Verification items for the finished model (mm, model axes). A direction names the side the tool comes from. Give positions to 0.01 mm unless a question says otherwise; leave off trailing zeros. Loops run counter-clockwise (first coordinate to the right, second up) from the corner with the lowest first, then second, coordinate; pieces in that order, holes last. Notation, with made-up numbers: M -34.75,-10 L -9.75,-10 A31 cw -9.75,20 Z; hole C -40,-7 d1. An arc over 180 degrees is marked long. Use a Markdown table: item, result.
from build123d import *

# Parameters (mm, degrees)
BOSS_EXTRUDE1_DEPTH = 150
SKETCH2_W           = 12.7
SKETCH2_H           = 24.13
CUT_EXTRUDE1_DEPTH  = 156.216502449
SKETCH3_W           = 149.993973466
SKETCH3_H           = 14.75620072
BOSS_EXTRUDE2_DEPTH = 3.55599999
SKETCH4_W           = 3.55599999
SKETCH4_H           = 13.202768596
CUT_EXTRUDE2_DEPTH  = 152.137564539
DRAFT1_START        = -153.930973466
DRAFT1_DEPTH        = 149.993973466
DRAFT2_START        = -153.937
DRAFT2_DEPTH        = 150
FILLET1_R           = 0.76200009
FILLET2_R           = 1.98120009
FILLET3_R           = 2.54


# Read off the part's stored shape, not the designer's step: Draft1, Draft2
with BuildPart() as part:
    # Sketch1 → Boss-Extrude1 (new body)
    with BuildSketch(Plane(origin=(-3.937, 0, 0), x_dir=(0, 0, -1), z_dir=(1, 0, 0))):
        with BuildLine():
            Line((2.311399989, 16.37657286), (2.311399989, -16.37657286))
            ThreePointArc((2.311399989, -16.37657286), (0.354826715, -15.481038557), (-1.770730805, -15.815950332))
            ThreePointArc((-1.770730805, -15.815950332), (-3.400639082, -15.955235788), (-4.710462095, -14.975253591))
            Line((-4.710462095, -14.975253591), (-5.7404, -15.627692517))
            ThreePointArc((-5.7404, -15.627692517), (-3.73586423, -17.127444277), (-1.241474216, -16.914283663))
            ThreePointArc((-1.241474216, -16.914283663), (0.188944014, -16.688900954), (1.505642365, -17.291560998))
            ThreePointArc((1.505642365, -17.291560998), (2.81343034, -17.487614789), (3.53059999, -16.37657286))
            Line((3.53059999, -16.37657286), (3.53059999, 16.37657286))
            ThreePointArc((3.53059999, 16.37657286), (2.81343034, 17.487614789), (1.505642365, 17.291560998))
            ThreePointArc((1.505642365, 17.291560998), (0.188944014, 16.688900954), (-1.241474216, 16.914283663))
            ThreePointArc((-1.241474216, 16.914283663), (-3.73586423, 17.127444277), (-5.7404, 15.627692517))
            Line((-5.7404, 15.627692517), (-4.710462095, 14.975253591))
            ThreePointArc((-4.710462095, 14.975253591), (-3.400639082, 15.955235788), (-1.770730805, 15.815950332))
            ThreePointArc((-1.770730805, 15.815950332), (0.354826715, 15.481038557), (2.311399989, 16.37657286))
        make_face()
    extrude(amount=-BOSS_EXTRUDE1_DEPTH)

    # Sketch2 → Cut-Extrude1 (cut, through all)
    with BuildSketch(Plane(origin=(0, 0, -3.53059999), x_dir=(-1, 0, 0), z_dir=(0, 0, -1))):
        with Locations((10.287, 0)):
            Rectangle(SKETCH2_W, SKETCH2_H)
    extrude(amount=-CUT_EXTRUDE1_DEPTH, mode=Mode.SUBTRACT)

    # Sketch3 → Boss-Extrude2 (add)
    with BuildSketch(Plane.XY.offset(-2.311399989)):
        with Locations((-78.933986733, 0)):
            Rectangle(SKETCH3_W, SKETCH3_H)
    extrude(amount=BOSS_EXTRUDE2_DEPTH)

    # Sketch4 → Cut-Extrude2 (cut, through all)
    with BuildSketch(Plane.ZY.offset(153.937)):
        with Locations((-1.752599995, 0)):
            Rectangle(SKETCH4_W, SKETCH4_H)
    extrude(amount=-CUT_EXTRUDE2_DEPTH, mode=Mode.SUBTRACT)

    # Draft1 outline → Draft1 (add)
    with BuildSketch(Plane.YZ.offset(DRAFT1_START)):
        Polygon((7.37810036, 1.244600001), (7.37810036, -2.311399989), (9.036290388, -2.311399989), align=None)
        Polygon((-7.37810036, 1.244600001), (-9.036290388, -2.311399989), (-7.37810036, -2.311399989), align=None)
    extrude(amount=DRAFT1_DEPTH)

    # Draft2 outline → Draft2 (cut)
    with BuildSketch(Plane.YZ.offset(DRAFT2_START)):
        Polygon((6.601384298, 0.0254), (6.601384298, -3.53059999), (8.259574326, -3.53059999), align=None)
        Polygon((-8.259574326, -3.53059999), (-6.601384298, -3.53059999), (-6.601384298, 0.0254), align=None)
    extrude(amount=DRAFT2_DEPTH, mode=Mode.SUBTRACT)

    # Fillet1
    fillet1_edges = [part.edges().sort_by_distance(p)[0] for p in [
        (-85.283986733, -9.036290388, -2.311399989),
        (-85.283986733, 9.036290388, -2.311399989),
        (-78.933986733, 6.601384298, 0.0254),
        (-78.933986733, -6.601384298, 0.0254),
    ]]
    fillet(fillet1_edges, radius=FILLET1_R)

    # Fillet2
    fillet2_edges = [part.edges().sort_by_distance(p)[0] for p in [
        (-78.933986733, -7.37810036, 1.244600001),
        (-78.933986733, 7.37810036, 1.244600001),
        (-85.287, -8.259574326, -3.53059999),
        (-85.287, 8.259574326, -3.53059999),
    ]]
    fillet(fillet2_edges, radius=FILLET2_R)

    # Fillet3
    fillet3_edges = [part.edges().sort_by_distance(p)[0] for p in [
        (-16.637, 12.065, -2.92099999),
        (-16.637, -12.065, -2.92099999),
    ]]
    fillet(fillet3_edges, radius=FILLET3_R)


solid = part.part
(1) Draft check along Y on faces 1 (the cylindrical face through (-77.887, 15.477, -0.325)), 2 (the cylindrical face through (-77.887, 17.137, 3.701)), 3 (the flat face through (-3.937, -0.1, 0.3)), 4 (the flat face through (-78, 13, -2.311)). Enter one of: +Y half, -Y half, draft (parallel to the pull), parting line (faces both ways), or undercut.
Results below:
| item | result |
|---|---|
| face 1 | undercut |
| face 2 | +Y half |
| face 3 | draft |
| face 4 | undercut |
(2) Set-up check for faces 5 (the flat face through (-80, 0, 1.245)), 6 (the cylindrical face through (-77.89, 15.95, 3.42)), 7 (the cylindrical face through (-15.913, 11.301, -2.912)): record each of +Z, -Z, +X, -X, +Y, -Y from which the full face is reachable in a straight line by a thin tool's end or side.
Results below:
| item | result |
|---|---|
| face 5 | +Z, +X, -X |
| face 6 | +X, -X |
| face 7 | +Z, -Z, +X |
(3) Cross-section at B-B on y = -4. Record the cut outline in (x, z).
Results below:
| item | result |
|---|---|
| outline | M -153.93,0.03 L -3.94,0.03 L -3.94,1.24 L -153.93,1.24 Z |
(4) Cross-section at A-A on z = 3.25. Record the cut outline in (x, y).
Results below:
| item | result |
|---|---|
| outline | M -153.94,-17.23 L -3.94,-17.23 L -3.94,-15.99 L -153.94,-15.99 Z; M -153.94,15.99 L -3.94,15.99 L -3.94,17.23 L -153.94,17.23 Z |
(5) Material ranges on line 1 (Y direction, x = -106.5, z = -1.75); line 2 (Y direction, x = -144, z = -0.5); line 3 (Y direction, x = -30.5, z = 4.75), recorded low to high.
Results below:
| item | result |
|---|---|
| line 1 | -17.46 to -15.97, -8.77 to -7.43, 7.43 to 8.77, 15.97 to 17.46 |
| line 2 | -16.75 to -15.5, -8.19 to -6.85, 6.85 to 8.19, 15.5 to 16.75 |
| line 3 | -16.65 to -15, 15 to 16.65 |
(6) Gauge pin test, flat ends, axial feed: P1, Ø6, axis at x = -102.5, y = -3, coming from the -Z side; P2, Ø6, axis at x = -63.5, y = 5, coming from the +Z side; P3, Ø3, axis at x = -26.5, z = 3.5, coming from the -Y side; P4, Ø0.6, axis at x = -10, z = -2.5, coming from the +Y side. Record the tip position at first contact, or that the pin passes through.
Results below:
| item | result |
|---|---|
| P1 | z = 0.03 |
| P2 | z = 1.24 |
| P3 | y = -17.26 |
| P4 | y = 17.6 |
